Here's how the part is built. I have some questions about the finished solid (model axes, mm). A direction names the side the tool comes from. Round coordinates to 2 decimals unless told otherwise and drop trailing zeros. Order: outer loops, then holes, each group sorted by start corner. A loop starts at its lowest first (then second) coordinate and runs counter-clockwise, first axis right, second up. Notation, with made-up numbers: (-37.5, -16) -> (-10.5, -16) arc R17 ccw to (-10.5, -9) -> close; hole circle Ø6 at (-36, 63.5). An arc over 180 degrees is marked (long way). Use a Markdown table: item, result. Add a question column.
(1) I want a section at B-B, the plane z = 43.75. Please give me the cut outline in (x, y).
(2) I'm going to push flat-ended pins straight in: P1, Ø10, axis at x = -63.43, y = -63.2, coming from the +Z side; P2, Ø3.5, axis at y = -27.5, z = 47.5, coming from the -X side; P3, Ø20, axis at x = -51.5, y = -25, coming from the +Z side; P4, Ø3, axis at x = 0.5, y = -46.5, coming from the -Z side. Where does each tip first touch, or does it pass through?
(3) I want a section at A-A, the plane y = -53.5. Please give me the cut outline in (x, z), then the cut area to 3 significant figures.
(4) I want a section at C-C, the plane z = 37.25. Please give me the cut outline in (x, y), then the cut area to 3 significant figures.
(5) I want a section at D-D, the plane x = 6. Please give me the cut outline in (y, z), then the cut area to 3 significant figures.
(6) Thinking about a two-plate mould opening in X: for faces 1 (the face through (-72.51, -72.38, 40.61)), 2 (the face through (50, -38, 45.508)), 3 (the face through (63.28, -9.46, 40.61)), which applies, pulls with the +X half, pulls with the -X half, needs draft (parallel to the pull), parting line crosses it, or undercut?
(7) On a 3-axis mill with a long thin cutter (end or side, diameter ignored), from which of +Z, -Z, +X, -X, +Y, -Y can I reach the whole of each face in a straight line? I mean faces 4 (the face through (-76.128, -38, 41)), 5 (the face through (30.298, -38, 38)), 6 (the face through (-56, -38, 45.508)), 7 (the face through (50, -38, 35.856)), 8 (the face through (30.298, -38, 47)). Say none if no direction works.
(8) If I drill on probe 1 along X at (y, z) = (-14.5, 42); probe 2 along X at (y, z) = (-64, 41.25); probe 3 along Y at (x, z) = (-58, 38.5), over which ranges is the centre line in solid material (lowest first)?
from build123d import *

# Parameters (mm, degrees)
F1_DEPTH = 76.2
F2_R     = 12.7
F3_R     = 6.35
F4_DEPTH = 48.811145


with BuildPart() as f1:
    # F0 (on Front) → F1 (new body)
    with BuildSketch(Plane.XZ):
        Polygon((-36.504163, 45.508145), (-76.128163, 45.508145), (-76.128163, 35.856145), (-36.504163, 35.856145), (-36.504163, 39.158145), (30.297837, 39.158145), (30.297837, 35.856145), (69.921837, 35.856145), (69.921837, 45.508145), (30.297837, 45.508145), (30.297837, 48.810145), (-36.504163, 48.810145), align=None)
    extrude(amount=F1_DEPTH)

    # F2
    f2_edges = [f1.edges().sort_by_distance(p)[0] for p in [
        (69.921837, 0, 40.682145),
        (69.921837, -76.2, 40.682145),
        (-76.128163, -76.2, 40.682145),
        (-76.128163, 0, 40.682145),
    ]]
    fillet(f2_edges, radius=F2_R)

    # F3 (on Top) → F4 (cut, through all)
    with BuildSketch(Plane.XY):
        with Locations((57.221837, -11.364109)):
            Circle(F3_R)
        with Locations((57.221837, -63.199298)):
            Circle(F3_R)
        with Locations((-63.428163, -63.199298)):
            Circle(F3_R)
        with Locations((-63.428163, -11.364109)):
            Circle(F3_R)
    extrude(amount=F4_DEPTH, mode=Mode.SUBTRACT)


solid = f1.part
Taken from the geometry:
| question | item | result |
|---|---|---|
| 1 | outline | (-76.13, -63.5) arc R12.7 ccw to (-63.43, -76.2) -> (57.22, -76.2) arc R12.7 ccw to (69.92, -63.5) -> (69.92, -12.7) arc R12.7 ccw to (57.22, 0) -> (-63.43, 0) arc R12.7 ccw to (-76.13, -12.7) -> close; hole circle Ø12.7 at (-63.43, -63.2); hole circle Ø12.7 at (-63.43, -11.36); hole circle Ø12.7 at (57.22, -63.2); hole circle Ø12.7 at (57.22, -11.36) |
| 2 | P1 | passes through |
| 2 | P2 | stops at x = -36.5 |
| 2 | P3 | stops at z = 45.51 |
| 2 | P4 | stops at z = 39.16 |
| 3 | outline | (-76.13, 35.86) -> (-36.5, 35.86) -> (-36.5, 39.16) -> (30.3, 39.16) -> (30.3, 35.86) -> (69.92, 35.86) -> (69.92, 45.51) -> (30.3, 45.51) -> (30.3, 48.81) -> (-36.5, 48.81) -> (-36.5, 45.51) -> (-76.13, 45.51) -> close |
| 3 | area | 1,410 mm2 |
| 4 | outline | (-76.13, -63.5) arc R12.7 ccw to (-63.43, -76.2) -> (-36.5, -76.2) -> (-36.5, 0) -> (-63.43, 0) arc R12.7 ccw to (-76.13, -12.7) -> close; (30.3, -76.2) -> (57.22, -76.2) arc R12.7 ccw to (69.92, -63.5) -> (69.92, -12.7) arc R12.7 ccw to (57.22, 0) -> (30.3, 0) -> close; hole circle Ø12.7 at (-63.43, -63.2); hole circle Ø12.7 at (-63.43, -11.36); hole circle Ø12.7 at (57.22, -63.2); hole circle Ø12.7 at (57.22, -11.36) |
| 4 | area | 5,390 mm2 |
| 5 | outline | (-76.2, 39.16) -> (0, 39.16) -> (0, 48.81) -> (-76.2, 48.81) -> close |
| 5 | area | 735 mm2 |
| 6 | face 1 | pulls with the -X half |
| 6 | face 2 | needs draft |
| 6 | face 3 | undercut |
| 7 | face 4 | +Z, -Z, -X, +Y, -Y |
| 7 | face 5 | -Z, +Y, -Y |
| 7 | face 6 | +Z, -X, +Y, -Y |
| 7 | face 7 | -Z, +X, -X, +Y, -Y |
| 7 | face 8 | +Z, +X, +Y, -Y |
| 8 | probe 1 | x = -76.13 to -68.95, -57.91 to 51.7, 62.74 to 69.92 |
| 8 | probe 2 | x = -76.12 to -69.73, -57.13 to 50.92, 63.52 to 69.91 |
| 8 | probe 3 | y = -76.2 to -66.49, -59.9 to -14.66, -8.07 to 0 |
